Build history of the part. All positions in model axes, mm. A direction names the side the tool comes from. Give positions to 0.01 mm unless a question says otherwise; leave off trailing zeros. Write each loop counter-clockwise with the first axis right and the second up, starting at its lowest first coordinate (ties: lowest second). Pieces come first, ordered by that corner, then holes. Notation, with made-up numbers: (59.25, 27) -> (91.25, 27) arc R22 ccw to (91.25, 59) -> close; hole circle Ø7 at (87.25, 86). An arc over 180 degrees is marked (long way). One line per question, with ' | ' between items. Start each with the question number.
(1) Pull direction Y, two halves, no side cores. Call faces 6 (the flat face through (0, -4, 9.824)), 7 (the conical face through (-0.14, -25.18, 3.3)), 8 (the cylindrical face through (0.038, -43.655, 2.993)), 9 (the cylindrical face through (0.04, -1.11, 2.99)): released by +Y, released by -Y, zero draft, split by the parting line, or undercut.
(2) Band-saw the part on D-D, the plane x = -0.5. Count the separate pieces of the cut face and the enclosed holes in it, and give its area (3 significant figures).
(3) Pin check, flat tips, straight feed: P1, Ø3, axis at x = 0, z = 6.98, coming from the -Y side; P2, Ø4.5, axis at x = 1, z = 6, coming from the -Y side; P3, Ø2.5, axis at x = 0.5, z = 6, coming from the -Y side; P4, Ø0.6, axis at y = -16.5, z = -0.5, coming from the -X side. Stop position of each tip, or through.
(4) Band-saw the part on B-B, the plane y = -36.5. Give the cut face in (x, z).
(5) Drill centre lines: probe 1 along Y at (x, z) = (0, 1.05); probe 2 along Y at (x, z) = (2.5, 2.75); probe 3 along X at (y, z) = (-4, 7). Where is each one in solid material? Low to high. Write a range as from..to.
(6) Band-saw the part on C-C, the plane z = 2. Give the cut face in (x, y).
(7) Band-saw the part on A-A, the plane y = -17. Give the cut face in (x, z), and give its area (3 significant figures).
(8) Tool access for faces 1 (the cylindrical face through (-0.04, -22.38, 2.99)), 2 (the flat face through (-3, -25, -2.54)), 3 (the flat face through (-2.718, -25, 5)), 4 (the flat face through (-5.863, -25, -2)), 5 (the flat face through (4.07, -25, -1)): list every direction of +Z, -Z, +X, -X, +Y, -Y with a clear straight run to the whole face (end or side of a thin tool).
from build123d import *

# Parameters (mm, degrees)
SKETCH1_W                            = 5.4356
SKETCH1_H                            = 5.08
BOSS_EXTRUDE1_DEPTH                  = 50.8
SKETCH4_W                            = 5.4356
SKETCH4_H                            = 7.283958
BOSS_EXTRUDE3_DEPTH                  = 5.08
SKETCH13_W                           = 7.283958
SKETCH13_H                           = 5.08
BOSS_EXTRUDE6_DEPTH                  = 5.4356
FILLET1_R                            = 1.5875
F_4_CLEARANCE_HOLE1_D                = 3.4544
FILLET1_OF_MIRROR5_R                 = 1.5875
BOSS_EXTRUDE4_DEPTH                  = 50.8
TAPPED_HOLE_FOR_4_40_HELICOIL1_D     = 3.048
TAPPED_HOLE_FOR_4_40_HELICOIL1_DEPTH = 5.08
TAPPED_HOLE_FOR_4_40_HELICOIL1_TIP   = 0.915711583


with BuildPart() as part:
    # Sketch1 → Boss-Extrude1 (new body)
    with BuildSketch(Plane(origin=(0, 0, 0), x_dir=(1, 0, 0), z_dir=(0, 1, 0))):
        Rectangle(SKETCH1_W, SKETCH1_H)
    extrude(amount=-BOSS_EXTRUDE1_DEPTH)

    # Sketch4 → Boss-Extrude3 (add)
    with BuildSketch(Plane(origin=(0, -1.5875, 0), x_dir=(1, 0, 0), z_dir=(0, 1, 0))):
        with Locations((0, -6.181979)):
            Rectangle(SKETCH4_W, SKETCH4_H)
    boss_extrude3 = extrude(amount=-BOSS_EXTRUDE3_DEPTH)

    # Sketch13 → Boss-Extrude6 (add)
    with BuildSketch(Plane(origin=(2.7178, 0, 0), x_dir=(0, 0, -1), z_dir=(1, 0, 0))):
        with Locations((-6.181979, -25.4)):
            Rectangle(SKETCH13_W, SKETCH13_H)
    extrude(amount=-BOSS_EXTRUDE6_DEPTH)

    # Fillet1
    fillet1_edges = [part.edges().sort_by_distance(p)[0] for p in [
        (0, -6.6675, 2.54),
        (0, -1.5875, 2.54),
        (0, -27.94, 2.54),
        (0, -22.86, 2.54),
    ]]
    fillet(fillet1_edges, radius=FILLET1_R - 0.0001)  # a hair under: the kernel refuses the full size

    # #4 Clearance Hole1 (through all)
    with Locations(Plane(origin=(0, 0, 0), x_dir=(1, 0, 0), z_dir=(0, 1, 0))):
        with Locations((0, -6.975729)):
            f_4_clearance_hole1 = Hole(F_4_CLEARANCE_HOLE1_D / 2)

    # Mirror5: Boss-Extrude3, #4 Clearance Hole1 across plane
    add(boss_extrude3.mirror(Plane.ZX.offset(-25.4)))
    add(f_4_clearance_hole1.mirror(Plane.ZX.offset(-25.4)), mode=Mode.SUBTRACT)

    # Fillet1 of Mirror5
    fillet1_of_mirror5_edges = [part.edges().sort_by_distance(p)[0] for p in [
        (0, -44.1325, 2.54),
        (0, -49.2125, 2.54),
        (0, -21.2726, 2.54),
        (0, -27.94, 4.1274),
    ]]
    fillet(fillet1_of_mirror5_edges, radius=FILLET1_OF_MIRROR5_R - 0.0001)  # a hair under: the kernel refuses the full size

    # Sketch7 → Boss-Extrude4 (add)
    with BuildSketch(Plane(origin=(0, 0, 0), x_dir=(1, 0, 0), z_dir=(0, 1, 0))):
        Polygon((3.207601712, -1.376528509), (3.207601712, 0.095381072), (4.069572105, 0.095381072), (4.069572105, 1.304918523), (5.863211288, 1.304918523), (5.863211288, 2.54), (2.7178, 2.54), (2.7178, -1.376528509), align=None)
    boss_extrude4 = extrude(amount=-BOSS_EXTRUDE4_DEPTH)

    # Mirror6: Boss-Extrude4 across plane
    add(boss_extrude4.mirror(Plane(origin=(0, 0, 0), x_dir=(0, 0, 1), z_dir=(1, 0, 0))))

    # Tapped Hole for #4-40 Helicoil1
    with Locations(Plane(origin=(0, 0, -2.54), x_dir=(-1, 0, 0), z_dir=(0, 0, -1))):
        with Locations((0, -4.1275), (0, -46.6725), (0, -25.4), (0, -14.76375), (0, -36.03625)):
            Hole(TAPPED_HOLE_FOR_4_40_HELICOIL1_D / 2, depth=TAPPED_HOLE_FOR_4_40_HELICOIL1_DEPTH)
            with Locations((0, 0, -(TAPPED_HOLE_FOR_4_40_HELICOIL1_DEPTH + TAPPED_HOLE_FOR_4_40_HELICOIL1_TIP / 2))):  # 118° drill point
                Cone(0, TAPPED_HOLE_FOR_4_40_HELICOIL1_D / 2, TAPPED_HOLE_FOR_4_40_HELICOIL1_TIP, mode=Mode.SUBTRACT)


solid = part.part
Results:
1) face 6: zero draft | face 7: undercut | face 8: undercut | face 9: released by +Y
2) separate pieces: 6 | enclosed holes: 0 | area: 246 mm²
3) P1: passes through | P2: stops at y = -49.26 | P3: stops at y = -49.21 | P4: stops at x = -4.07
4) outline: (-5.86, -2.54) -> (-1.45, -2.54) -> (-1.45, 2.54) -> (-2.72, 2.54) -> (-2.72, 1.38) -> (-3.21, 1.38) -> (-3.21, -0.1) -> (-4.07, -0.1) -> (-4.07, -1.3) -> (-5.86, -1.3) -> close; (1.45, -2.54) -> (5.86, -2.54) -> (5.86, -1.3) -> (4.07, -1.3) -> (4.07, -0.1) -> (3.21, -0.1) -> (3.21, 1.38) -> (2.72, 1.38) -> (2.72, 2.54) -> (1.45, 2.54) -> close
5) probe 1: y = -50.8..-48.2, -45.15..-37.56, -34.51..-26.92, -23.88..-16.29, -13.24..-5.65, -2.6..0 | probe 2: y = -50.01..-43.33, -28.74..-22.06, -7.47..-0.79 | probe 3: x = -2.72..-1.73, 1.73..2.72
6) outline: (-2.72, -50.8) -> (2.72, -50.8) -> (2.72, 0) -> (-2.72, 0) -> close; hole circle Ø3.05 at (0, -46.67); hole circle Ø3.05 at (0, -36.04); hole circle Ø3.05 at (0, -25.4); hole circle Ø3.05 at (0, -14.76); hole circle Ø3.05 at (0, -4.13)
7) outline: (-5.86, -2.54) -> (5.86, -2.54) -> (5.86, -1.3) -> (4.07, -1.3) -> (4.07, -0.1) -> (3.21, -0.1) -> (3.21, 1.38) -> (2.72, 1.38) -> (2.72, 2.54) -> (-2.72, 2.54) -> (-2.72, 1.38) -> (-3.21, 1.38) -> (-3.21, -0.1) -> (-4.07, -0.1) -> (-4.07, -1.3) -> (-5.86, -1.3) -> close | area: 40.1 mm²
8) face 1: +Z, +X, -X | face 2: -Z, +X, -X, +Y, -Y | face 3: +Z, -X, +Y, -Y | face 4: +Z, -Z, -X, +Y, -Y | face 5: +Z, +X, +Y, -Y
